Source: CAD feature listing. Evaluate the final solid. Frame: model axes, mm. A direction names the side the tool comes from. Round coordinates to 2 decimals unless told otherwise and drop trailing zeros. Loops run counter-clockwise (first coordinate to the right, second up) from the corner with the lowest first, then second, coordinate; pieces in that order, holes last.
(1) Set-up query: faces 1 (the flat face through (-238, -19, 1014)), 2 (the flat face through (1, -1, 0)). Return all of +Z, -Z, +X, -X, +Y, -Y with unobstructed straight access to the full face (end or side cutting, diameter ignored); none if empty.
(2) Material intervals for probe 1 along X at (y, z) = (-27.5, 1195); probe 2 along X at (y, z) = (-1.5, 1459); probe 3 along Y at (x, z) = (-108, 1521.5), sorted ascending.
(3) First-contact query: pin 1 Ø1.5 at (x, z) = (10.5, 1761.5) entering from -Y. Flat tip, straight axial feed; report the tip coordinate or a pass-through.
(4) Mould query, pull axis X, two halves, no side actions, for faces 3 (the flat face through (240, -19, 986)), 4 (the flat face through (-3, -2, 986)), 5 (the flat face through (-240, -19, 1014)), 6 (the flat face through (1, -1, 2000)). Classes: pulls with the +X half, pulls with the -X half, needs draft (parallel to the pull), parting line crosses it, or undercut.
(5) Section C-C, the plane x = -80. Return the cut outline in (y, z).
(6) Section A-A, the plane y = -17. Return the cut outline in (x, z).
(7) Section B-B, the plane z = 1719. Return the cut outline in (x, y), plus the area to 3 significant figures.
```python
from build123d import *

# Parameters (mm, degrees)
SKETCH1_W                      = 480
SKETCH1_H                      = 2
BASE_FLANGE1_DEPTH             = 2000
EDGE_FLANGE1_STRIP_W           = 9.4732
EDGE_FLANGE1_STRIP_H           = 2
EDGE_FLANGE1_STRIP_CUT_DEPTH   = 2000
EDGE_FLANGE1_STRIP_2_W         = 9.4732
EDGE_FLANGE1_STRIP_2_H         = 2
EDGE_FLANGE1_STRIP_CUT_2_DEPTH = 2000
EDGE_FLANGE1_DEPTH             = 2000
EDGE_FLANGE1_BEND_DEPTH        = 2000


# Sheet-metal steps are written as plain solids
with BuildPart() as part:
    # Sketch1 → Base-Flange1 (new body)
    with BuildSketch(Plane.XY):
        with Locations((0, -1)):
            Rectangle(SKETCH1_W, SKETCH1_H)
    extrude(amount=BASE_FLANGE1_DEPTH)

    # Edge-Flange1 strip (across the edge) → Edge-Flange1 strip cut (cut)
    with BuildSketch(Plane(origin=(240, -2, 0), x_dir=(-1, 0, 0), z_dir=(0, 0, 1))):
        with Locations((-2, -1)):
            Rectangle(EDGE_FLANGE1_STRIP_W, EDGE_FLANGE1_STRIP_H)
    extrude(amount=EDGE_FLANGE1_STRIP_CUT_DEPTH, mode=Mode.SUBTRACT)

    # Edge-Flange1 strip 2 (across the edge) → Edge-Flange1 strip cut 2 (cut)
    with BuildSketch(Plane(origin=(-240, -2, 2000), x_dir=(1, 0, 0), z_dir=(0, 0, -1))):
        with Locations((-2, -1)):
            Rectangle(EDGE_FLANGE1_STRIP_2_W, EDGE_FLANGE1_STRIP_2_H)
    extrude(amount=EDGE_FLANGE1_STRIP_CUT_2_DEPTH, mode=Mode.SUBTRACT)

    # Edge-Flange1 section (across the edge) → Edge-Flange1 (add)
    with BuildSketch(Plane(origin=(240, -2, 0), x_dir=(-1, 0, 0), z_dir=(0, 0, 1))):
        with BuildLine():
            Line((0, 0.7366), (0, 33))
            Line((0, 33), (2, 33))
            Line((2, 33), (2, 0.7366))
            ThreePointArc((2, 0.7366), (2.215745145, 0.215745145), (2.7366, 0))
            Line((2.7366, 0), (2.7366, -2))
            ThreePointArc((2.7366, -2), (0.801531583, -1.198468417), (0, 0.7366))
        make_face()
    extrude(amount=EDGE_FLANGE1_DEPTH)

    # Edge-Flange1 section 2 (across the edge) → Edge-Flange1 bend (add)
    with BuildSketch(Plane(origin=(-240, -2, 2000), x_dir=(1, 0, 0), z_dir=(0, 0, -1))):
        with BuildLine():
            Line((0, 0.7366), (0, 33))
            Line((0, 33), (2, 33))
            Line((2, 33), (2, 0.7366))
            ThreePointArc((2, 0.7366), (2.215745145, 0.215745145), (2.7366, 0))
            Line((2.7366, 0), (2.7366, -2))
            ThreePointArc((2.7366, -2), (0.801531583, -1.198468417), (0, 0.7366))
        make_face()
    extrude(amount=EDGE_FLANGE1_BEND_DEPTH)


solid = part.part
```
Output values:
1. face 1: +Z, -Z, -Y
1. face 2: -Z, +X, -X, +Y, -Y
2. probe 1: x = -240 to -238, 238 to 240
2. probe 2: x = -239.7 to 239.7
2. probe 3: y = -2 to 0
3. pin 1: stops at y = -2
4. face 3: pulls with the +X half
4. face 4: undercut
4. face 5: pulls with the -X half
4. face 6: needs draft
5. outline: (-2, 0) - (0, 0) - (0, 2000) - (-2, 2000) - close
6. outline: (-240, 0) - (-238, 0) - (-238, 2000) - (-240, 2000) - close; (238, 0) - (240, 0) - (240, 2000) - (238, 2000) - close
7. outline: (-240, -35) - (-238, -35) - (-238, -2.74) arc R0.74 cw to (-237.26, -2) - (237.26, -2) arc R0.74 cw to (238, -2.74) - (238, -35) - (240, -35) - (240, -2.74) arc R2.74 ccw to (237.26, 0) - (-237.26, 0) arc R2.74 ccw to (-240, -2.74) - close
7. area: 1,090 mm2
